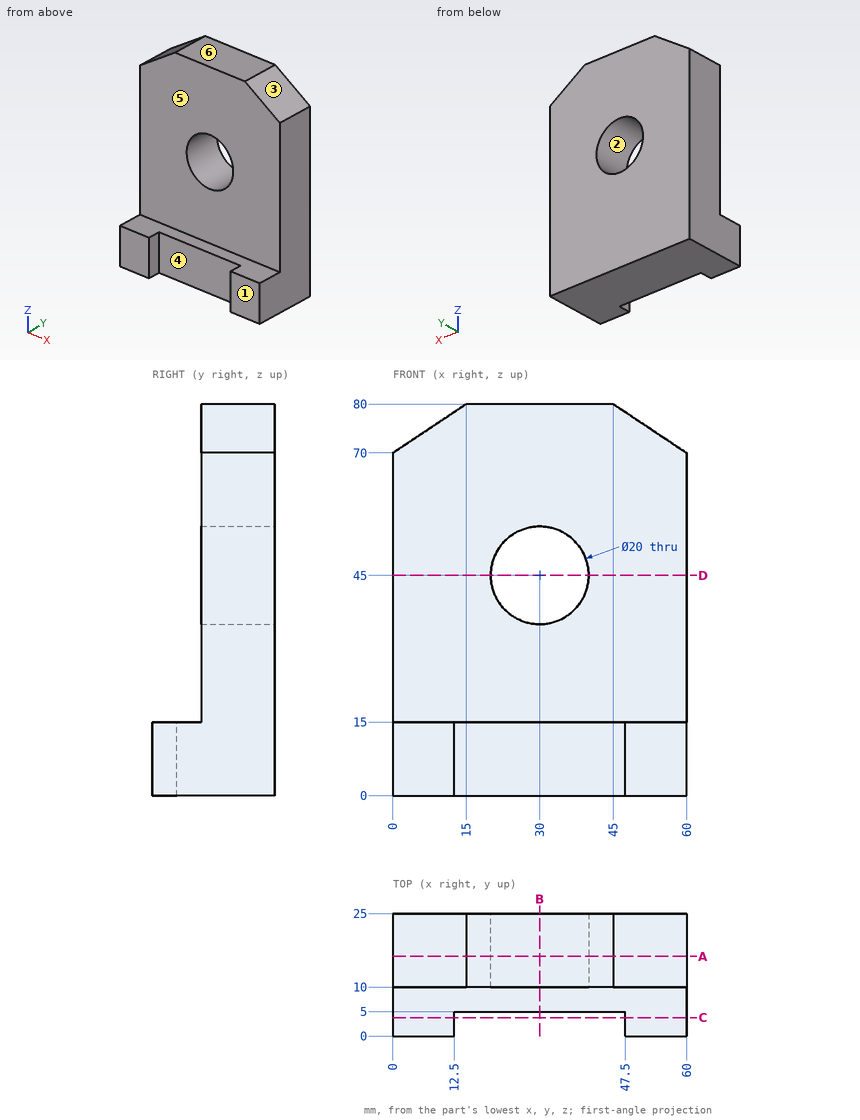
Here's the drawing with two shaded views (mm, measured from the low corner). I have some questions. A direction names the side the tool comes from. Round coordinates to 2 decimals unless told otherwise and drop trailing zeros. Loops run counter-clockwise (first coordinate to the right, second up) from the corner with the lowest first, then second, coordinate; pieces in that order, holes last. Notation, with made-up numbers: (84, -17.75) -> (133, -17.75) arc R14 cw to (133, 6.25) -> close; hole circle Ø1 at (68, 51). An arc over 180 degrees is marked (long way). Answer as CSV lines item,"result". Start each with the question number.
1. I need wall thicknesses on probe 1 along X at (y, z) = (15.5, 45); probe 2 along Z at (x, y) = (30, 13.5); probe 3 along Z at (x, y) = (12.5, 6.5). Which ranges of each line are inside material? Lowest first, please. Write a range as from..to.
2. Imagine slicing it at B-B on x = 30. Write out the boundary of the cut face in (y, z).
3. If we mould it in two halves opening along Z, with no side actions, what happens to the marked faces 1, 2 and 3? For each: pulls with the +Z half, pulls with the -Z half, needs draft (parallel to the pull), parting line crosses it, or undercut.
4. I'm going to push flat-ended pins straight in: P1, Ø4.5, axis at x = 32, z = 8.5, coming from the -Y side; P2, Ø8, axis at x = 23, z = 29.5, coming from the -Y side; P3, Ø2, axis at x = 10.5, y = 13.5, coming from the +Z side. Where does each tip first touch, or does it pass through?
5. Imagine slicing it at A-A on y = 16.25. Write out the boundary of the cut face in (x, z), plus the area to 3 significant figures.
6. For the marked faces 4, 5 and 6, which set-ups out of +Z, -Z, +X, -X, +Y, -Y let a thin tool reach every point of the face, with its end or its side?
7. Imagine slicing it at D-D on z = 45. Write out the boundary of the cut face in (x, y), plus the area to 3 significant figures.
8. Imagine slicing it at C-C on y = 3.75. Write out the boundary of the cut face in (x, z).
Solution:
1,probe 1,"0..20, 40..60"
1,probe 2,"0..35, 55..80"
1,probe 3,"0..15"
2,outline,"(5, 0) -> (25, 0) -> (25, 35) -> (10, 35) -> (10, 15) -> (5, 15) -> close; (10, 55) -> (25, 55) -> (25, 80) -> (10, 80) -> close"
3,face 1,"needs draft"
3,face 2,"undercut"
3,face 3,"pulls with the +Z half"
4,P1,"y = 5"
4,P2,"y = 10"
4,P3,"z = 77.67"
5,outline,"(0, 0) -> (60, 0) -> (60, 70) -> (45, 80) -> (15, 80) -> (0, 70) -> close; hole circle Ø20 at (30, 45)"
5,area,"4,340 mm²"
6,face 4,"+Z, -Z, -Y"
6,face 5,"+Z, +X, -X, -Y"
6,face 6,"+Z, +X, -X, +Y, -Y"
7,outline,"(0, 10) -> (20, 10) -> (20, 25) -> (0, 25) -> close; (40, 10) -> (60, 10) -> (60, 25) -> (40, 25) -> close"
7,area,"600 mm²"
8,outline,"(0, 0) -> (12.5, 0) -> (12.5, 15) -> (0, 15) -> close; (47.5, 0) -> (60, 0) -> (60, 15) -> (47.5, 15) -> close"
